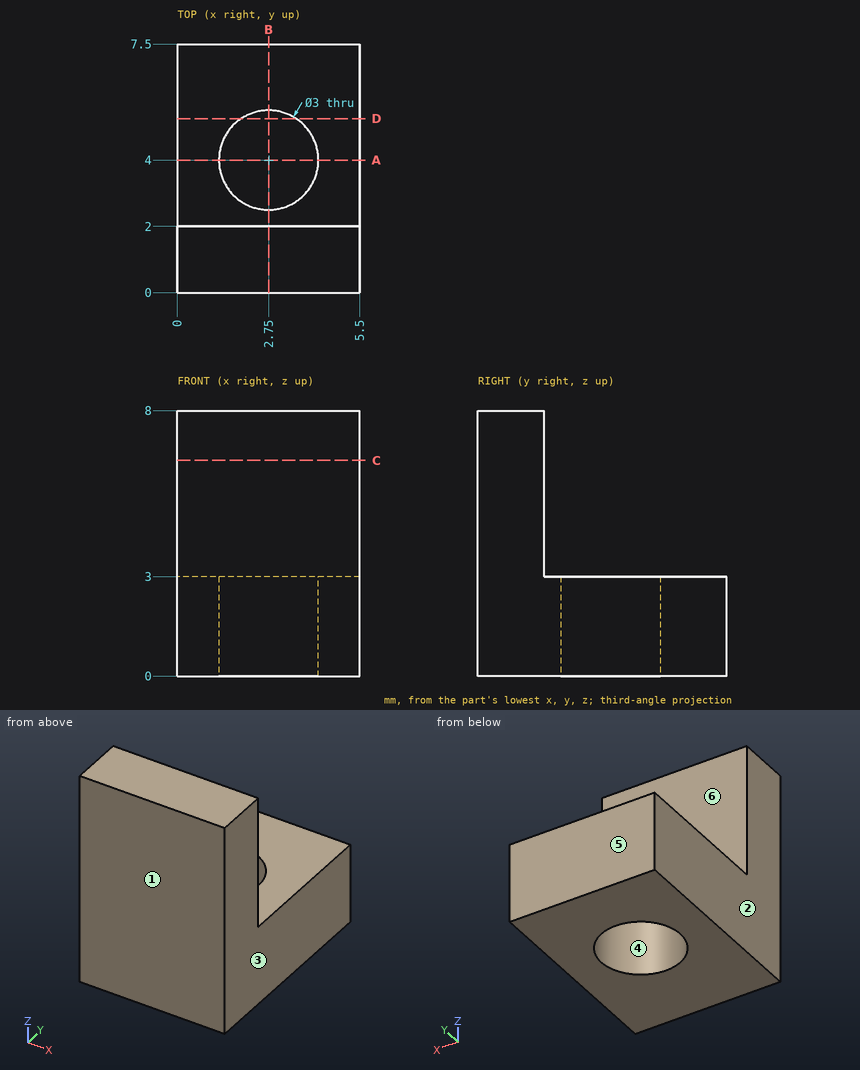
Geometry: see drawing. Coordinates: mm, zero at the bounding-box minimum. A direction names the side the tool comes from. Give positions to 0.01 mm unless a question says otherwise; leave off trailing zeros. Order: outer loops, then holes, each group sorted by start corner. A loop starts at its lowest first (then second) coordinate and runs counter-clockwise, first axis right, second up. Notation, with made-up numbers: (88, 57.25) -> (97, 57.25) arc R29 ccw to (97, 94.25) -> close; hole circle Ø10 at (86, 38). An arc over 180 degrees is marked (long way). Write each question's results on one line, items separated by ' | '.
1) Cut plane B-B (x = 2.75). Output: boundary loops of the cut face in (y, z).
Geometry says:
outline: (0, 0) -> (2.5, 0) -> (2.5, 3) -> (2, 3) -> (2, 8) -> (0, 8) -> close; (5.5, 0) -> (7.5, 0) -> (7.5, 3) -> (5.5, 3) -> close
2) Draft query along X for the marked faces 1, 2, 3 and 4. Return one class per face: released by +X, released by -X, zero draft, split by the parting line, or undercut.
Geometry says:
face 1: zero draft | face 2: released by -X | face 3: released by +X | face 4: undercut
3) Line query: line 1 along Y through (x, z) = (2.75, 1.7); line 2 along Y through (x, z) = (4.15, 3.25); line 3 along Z through (x, y) = (4.6, 4.25). Output: solid intervals per line, ascending.
Geometry says:
line 1: y = 0 to 2.5, 5.5 to 7.5 | line 2: y = 0 to 2 | line 3: z = 0 to 3
4) Cut plane D-D (y = 5.25). Output: boundary loops of the cut face in (x, z), and give its area (3 significant figures).
Geometry says:
outline: (0, 0) -> (1.92, 0) -> (1.92, 3) -> (0, 3) -> close; (3.58, 0) -> (5.5, 0) -> (5.5, 3) -> (3.58, 3) -> close | area: 11.5 mm²
5) Cut plane C-C (z = 6.5). Output: boundary loops of the cut face in (x, y).
Geometry says:
outline: (0, 0) -> (5.5, 0) -> (5.5, 2) -> (0, 2) -> close
6) First-contact query: pin 1 Ø3 at (x, y) = (1.5, 5) entering from +Z. Flat tip, straight axial feed; report the tip coordinate or a pass-through.
Geometry says:
pin 1: stops at z = 3
7) Set-up query: the marked faces 5 and 6. Return all of +Z, -Z, +X, -X, +Y, -Y with unobstructed straight access to the full face (end or side cutting, diameter ignored); none if empty.
Geometry says:
face 5: +Z, -Z, +X, -X, +Y | face 6: +Z, +X, -X, +Y
8) Cut plane A-A (y = 4). Output: boundary loops of the cut face in (x, z), and give its area (3 significant figures).
Geometry says:
outline: (0, 0) -> (1.25, 0) -> (1.25, 3) -> (0, 3) -> close; (4.25, 0) -> (5.5, 0) -> (5.5, 3) -> (4.25, 3) -> close | area: 7.50 mm²
